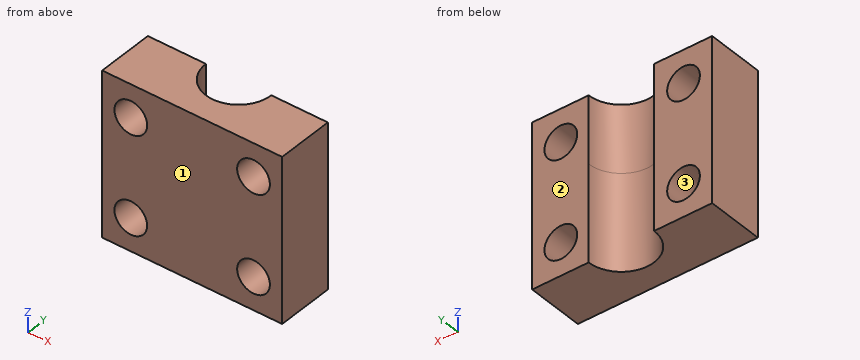
```python
from build123d import *

# Parameters (mm, degrees)
SKETCH1_W                      = 44
SKETCH1_H                      = 40
SKETCH1_R                      = 4
BOSS_EXTRUDE1_DEPTH            = 14
CUT_EXTRUDE1_REACH             = 18.442
SKETCH2_R                      = 8
CUT_EXTRUDE1_DIRECTION_2_REACH = 25.558


with BuildPart() as part:
    # Sketch1 → Boss-Extrude1 (new body)
    with BuildSketch(Plane(origin=(0, 0, 0), x_dir=(1, 0, 0), z_dir=(0, 1, 0))):
        with Locations((-0.188936111, 3.557633072)):
            Rectangle(SKETCH1_W, SKETCH1_H)
        with Locations((14.811063889, -8.442366928)):
            Circle(SKETCH1_R, mode=Mode.SUBTRACT)
        with Locations((14.811063889, 15.557633072)):
            Circle(SKETCH1_R, mode=Mode.SUBTRACT)
        with Locations((-15.188936111, 15.557633072)):
            Circle(SKETCH1_R, mode=Mode.SUBTRACT)
        with Locations((-15.188936111, -8.442366928)):
            Circle(SKETCH1_R, mode=Mode.SUBTRACT)
    extrude(amount=BOSS_EXTRUDE1_DEPTH)

    # Cut-Extrude1: up to this face of the body (flat: up to its plane)
    cut_extrude1_end = Plane(part.part.faces().sort_by_distance((-0.188936111, 7, 16.442366928))[0])
    # Sketch2 → Cut-Extrude1 (cut, up to the picked face)
    with BuildSketch(Plane.XY, mode=Mode.PRIVATE) as cut_extrude1_sk1:
        with Locations((0, 14)):
            Circle(SKETCH2_R)
    cut_extrude1_tool1 = split(extrude(cut_extrude1_sk1.sketch, amount=CUT_EXTRUDE1_REACH, mode=Mode.PRIVATE), bisect_by=cut_extrude1_end, keep=Keep.BOTH, mode=Mode.PRIVATE)
    add(cut_extrude1_tool1.solids().sort_by_distance((0, 14, 0))[0], mode=Mode.SUBTRACT)

    # Cut-Extrude1 direction 2: up to this face of the body (flat: up to its plane)
    cut_extrude1_direction_2_end = Plane(part.part.faces().sort_by_distance((-0.188936111, 7, -23.557633072))[0])
    # Sketch2 → Cut-Extrude1 direction 2 (cut, up to the picked face)
    with BuildSketch(Plane.XY, mode=Mode.PRIVATE) as cut_extrude1_direction_2_sk1:
        with Locations((0, 14)):
            Circle(SKETCH2_R)
    cut_extrude1_direction_2_tool1 = split(extrude(cut_extrude1_direction_2_sk1.sketch, amount=-CUT_EXTRUDE1_DIRECTION_2_REACH, mode=Mode.PRIVATE), bisect_by=cut_extrude1_direction_2_end, keep=Keep.BOTH, mode=Mode.PRIVATE)
    add(cut_extrude1_direction_2_tool1.solids().sort_by_distance((0, 14, 0))[0], mode=Mode.SUBTRACT)


solid = part.part
```
Read the model definition and answer for the solid it produces. Units are mm, in the model's axes. Face numbers are marked on the shaded views. Coordinates: 2 decimals unless noted, no trailing zeros. Write each loop counter-clockwise with the first axis right and the second up, starting at its lowest first coordinate (ties: lowest second). Pieces come first, ordered by that corner, then holes. Notation, with made-up numbers: (28.5, 56) -> (74.5, 56) arc R11 ccw to (74.5, 64) -> close; hole circle Ø3 at (52, 27). An arc over 180 degrees is marked (long way). Return JSON: item names as keys, results as strings.
1. A cutting plane is placed at A-A (y = 13.25). Determine the outline of the cut face in (x, z), and give its area (3 significant figures).
Found:
{"outline": "(-22.19, -23.56) -> (-7.96, -23.56) -> (-7.96, 16.44) -> (-22.19, 16.44) -> close; (7.96, -23.56) -> (21.81, -23.56) -> (21.81, 16.44) -> (7.96, 16.44) -> close; hole circle Ø8 at (-15.19, -15.56); hole circle Ø8 at (-15.19, 8.44); hole circle Ø8 at (14.81, -15.56); hole circle Ø8 at (14.81, 8.44)", "area": "922 mm2"}
2. A cutting plane is placed at D-D (y = 9.5). Determine the outline of the cut face in (x, z).
Found:
{"outline": "(-22.19, -23.56) -> (-6.61, -23.56) -> (-6.61, 16.44) -> (-22.19, 16.44) -> close; (6.61, -23.56) -> (21.81, -23.56) -> (21.81, 16.44) -> (6.61, 16.44) -> close; hole circle Ø8 at (-15.19, -15.56); hole circle Ø8 at (-15.19, 8.44); hole circle Ø8 at (14.81, -15.56); hole circle Ø8 at (14.81, 8.44)"}
3. A cutting plane is placed at B-B (x = 15). Determine the outline of the cut face in (y, z), and give its area (3 significant figures).
Found:
{"outline": "(0, -23.56) -> (14, -23.56) -> (14, -19.55) -> (0, -19.55) -> close; (0, -11.56) -> (14, -11.56) -> (14, 4.45) -> (0, 4.45) -> close; (0, 12.44) -> (14, 12.44) -> (14, 16.44) -> (0, 16.44) -> close", "area": "336 mm2"}
4. Each of these flat-tipped pins is pushed along its axis until it touches: P1, Ø1, axis at x = -5.5, z = 9, coming from the +Y side; P2, Ø4, axis at x = 15.5, z = -19.5, coming from the -Y side; P3, Ø1.5, axis at x = -5.5, z = -17.5, coming from the +Y side. Where does it stop, or does it pass through?
Found:
{"P1": "y = 8.71", "P2": "y = 0", "P3": "y = 9.01"}
5. A cutting plane is placed at C-C (z = 2). Determine the outline of the cut face in (x, y), and give its area (3 significant figures).
Found:
{"outline": "(-22.19, 0) -> (21.81, 0) -> (21.81, 14) -> (8, 14) arc R8 cw to (-8, 14) -> (-22.19, 14) -> close", "area": "515 mm2"}
6. Find the intervals of material crossed by line 1 along Z through (x, y) = (15, 5.25); line 2 along X through (y, z) = (4.5, 9); line 3 along X through (y, z) = (10, -14), in increasing order. Write a range as from..to.
Found:
{"line 1": "-23.56..-19.55, -11.56..4.45, 12.44..16.44", "line 2": "-22.19..-19.15, -11.23..10.85, 18.77..21.81", "line 3": "-22.19..-18.87, -11.5..-6.93, 6.93..11.13, 18.5..21.81"}
7. Determine the mould class of the marked faces 1, 2 and 3 for opening direction Y: pulls with the +Y half, pulls with the -Y half, needs draft (parallel to the pull), parting line crosses it, or undercut.
Found:
{"face 1": "pulls with the -Y half", "face 2": "pulls with the +Y half", "face 3": "needs draft"}
